```python
from build123d import *

# Parameters (mm, degrees)
SKETCH1_R           = 3.8862
BOSS_EXTRUDE1_DEPTH = 12.7
SKETCH2_R           = 2.032
CUT_EXTRUDE1_DEPTH  = 2688.829818218
SKETCH3_R           = 2.032
CUT_EXTRUDE2_DEPTH  = 2688.975736213


with BuildPart() as part:
    # Sketch1 → Boss-Extrude1 (new body)
    with BuildSketch(Plane.XY):
        with BuildLine():
            Line((2687.674805049, 2686.446487648), (2687.674805049, 2660.523843887))
            Line((2687.674805049, 2660.523843887), (2548.863805049, 2660.523843887))
            Line((2548.863805049, 2660.523843887), (2548.863805049, 2700.62861103))
            Line((2548.863805049, 2700.62861103), (2535.274805049, 2700.62861103))
            Line((2535.274805049, 2700.62861103), (2535.274805049, 2702.662667964))
            add(Edge.make_bspline(
                [(2549.887954959, 2703.598313804), (2545.009565075, 2703.390230841), (2540.136123501, 2703.088635053), (2535.274805049, 2702.662667964)],
                knots=[10.93644372, 10.93644372, 10.93644372, 10.93644372, 11.514330156, 11.514330156, 11.514330156, 11.514330156], degree=3))
            ThreePointArc((2549.887954959, 2703.598313804), (2552.182411528, 2702.754004596), (2553.196580638, 2700.529403507))
            Line((2553.196580638, 2700.529403507), (2553.256507729, 2698.686786983))
            Line((2553.256507729, 2698.686786983), (2562.908507729, 2698.686786983))
            Line((2562.908507729, 2698.686786983), (2575.148807064, 2686.446487648))
            Line((2575.148807064, 2686.446487648), (2687.674805049, 2686.446487648))
        make_face()
        with Locations((2675.105839614, 2673.877522213)):
            Circle(SKETCH1_R, mode=Mode.SUBTRACT)
    extrude(amount=BOSS_EXTRUDE1_DEPTH)

    # Sketch2 → Cut-Extrude1 (cut, through all)
    with BuildSketch(Plane(origin=(0, 2686.446487648, 0), x_dir=(1, 0, 0), z_dir=(0, 1, 0))):
        with Locations(Location((2627.349805049, -6.35, 0), (0, 0, 180))):
            Circle(SKETCH2_R)
    extrude(amount=-CUT_EXTRUDE1_DEPTH, mode=Mode.SUBTRACT)

    # Sketch3 → Cut-Extrude2 (cut, through all)
    with BuildSketch(Plane(origin=(0, 2698.686786983, 0), x_dir=(1, 0, 0), z_dir=(0, 1, 0))):
        with Locations(Location((2558.082507729, -6.35, 0), (0, 0, 180))):
            Circle(SKETCH3_R)
    extrude(amount=-CUT_EXTRUDE2_DEPTH, mode=Mode.SUBTRACT)


solid = part.part
```
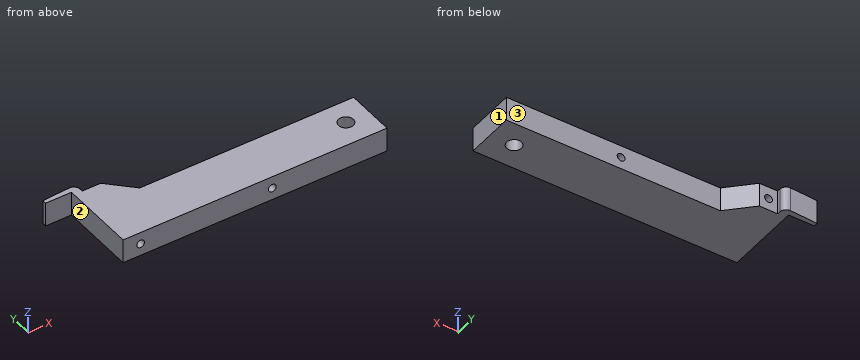
Can you work these out from the model? Positions are in its coordinate system, mm. Face numbers are marked on the shaded views. A direction names the side the tool comes from. Coordinates: 2 decimals unless noted, no trailing zeros. Loops run counter-clockwise (first coordinate to the right, second up) from the corner with the lowest first, then second, coordinate; pieces in that order, holes last. Notation, with made-up numbers: (85, 1.25) -> (130, 1.25) arc R7 cw to (130, 9.25) -> close; hole circle Ø7 at (-21, 11.25). An arc over 180 degrees is marked (long way). Put each result on its own line as item: value. Start each with the question number.
Q1. I'm going to push flat-ended pins straight in: P1, Ø3, axis at x = 2558.5, z = 4.5, coming from the +Y side; P2, Ø4, axis at x = 2664, z = 8.5, coming from the +Y side; P3, Ø2, axis at x = 2557, y = 2670.5, coming from the -Z side; P4, Ø6.5, axis at x = 2545, z = 4, coming from the -Y side. Where does each tip first touch, or does it pass through?
Q2. I want a section at C-C (y = 2690). Write out the boundary of the cut face in (x, z), plus the area to 3 significant figures.
Q3. I want a section at A-A (x = 2627.5). Write out the boundary of the cut face in (y, z).
Q4. I want a section at B-B (y = 2663.5). Write out the boundary of the cut face in (x, z).
Q5. For the marked faces 1, 2 and 3, which set-ups out of +Z, -Z, +X, -X, +Y, -Y let a thin tool reach every point of the face, with its end or its side?
Q6. I want a section at D-D (z = 6.35). Count the separate pieces of the cut face and the enclosed holes in it, plus the area to 3 significant figures.
Q7. If I drill on line 1 (X direction, y = 2684, z = 2); line 2 (X direction, y = 2665, z = 5.5); line 3 (Y direction, x = 2562, z = 8.75), over which ranges is the centre line in solid material (lowest first)? Write a range as [from, to].
Taken from the geometry:
1. P1: stops at y = 2698.69
1. P2: stops at y = 2686.45
1. P3: stops at z = 0
1. P4: stops at y = 2700.63
2. outline: (2548.86, 0) -> (2571.6, 0) -> (2571.6, 12.7) -> (2548.86, 12.7) -> close; hole circle Ø4.06 at (2558.08, 6.35)
2. area: 276 mm2
3. outline: (2660.52, 0) -> (2686.45, 0) -> (2686.45, 4.32) -> (2660.52, 4.32) -> close; (2660.52, 8.38) -> (2686.45, 8.38) -> (2686.45, 12.7) -> (2660.52, 12.7) -> close
4. outline: (2548.86, 0) -> (2687.67, 0) -> (2687.67, 12.7) -> (2548.86, 12.7) -> close; hole circle Ø4.06 at (2558.08, 6.35); hole circle Ø4.06 at (2627.35, 6.35)
5. face 1: +Z, -Z, +X, +Y, -Y
5. face 2: +Z, -Z, -X, -Y
5. face 3: +Z, -Z, +X, +Y
6. separate pieces: 3
6. enclosed holes: 1
6. area: 3,590 mm2
7. line 1: x = [2548.86, 2687.67]
7. line 2: x = [2548.86, 2556.24], [2559.93, 2625.5], [2629.2, 2687.67]
7. line 3: y = [2660.52, 2698.69]
